from build123d import *

# Parameters (mm, degrees)
BOSS_EXTRUDE1_DEPTH        = 76.2
SKETCH2_R                  = 38.1
BOSS_EXTRUDE2_DEPTH        = 12.7
F_3_4_1_5_DIAMETER_HOLE1_D = 38.1


with BuildPart() as part:
    # Sketch1 → Boss-Extrude1 (new body)
    with BuildSketch(Plane.XY):
        with BuildLine():
            ThreePointArc((0, 74.498522628), (-11.550198291, 75.086541233), (-18.788031752, 66.066196825))
            Line((-18.788031752, 66.066196825), (-31.095079379, 6.415492062))
            ThreePointArc((-31.095079379, 6.415492062), (-24.614572645, -20.054558422), (0, -31.75))
            Line((0, -31.75), (19.05, -31.75))
            Line((19.05, -31.75), (19.05, -44.45))
            Line((19.05, -44.45), (88.9, -44.45))
            Line((88.9, -44.45), (114.3, -25.4))
            Line((114.3, -25.4), (114.3, -12.7))
            Line((114.3, -12.7), (50.8, -12.7))
            Line((50.8, -12.7), (50.8, 0))
            Line((50.8, 0), (0, 0))
            Line((0, 0), (0, 74.498522628))
        make_face()
    extrude(amount=BOSS_EXTRUDE1_DEPTH)

    # Sketch2 → Boss-Extrude2 (add)
    with BuildSketch(Plane(origin=(0, -12.7, 0), x_dir=(1, 0, 0), z_dir=(0, 1, 0))):
        with Locations((50.8, -38.1)):
            Circle(SKETCH2_R)
    extrude(amount=BOSS_EXTRUDE2_DEPTH)

    # 3/4 (1.5) Diameter Hole1 (through all)
    with Locations(Plane(origin=(0, 0, 0), x_dir=(1, 0, 0), z_dir=(0, 1, 0))):
        with Locations((50.8, -38.1)):
            Hole(F_3_4_1_5_DIAMETER_HOLE1_D / 2)


solid = part.part
Could you check a few things on this model? Use its own coordinates, in mm. A direction names the side the tool comes from. Coordinates: 2 decimals unless noted, no trailing zeros. Order: outer loops, then holes, each group sorted by start corner. A loop starts at its lowest first (then second) coordinate and runs counter-clockwise, first axis right, second up. Notation, with made-up numbers: (17, -39.5) - (70, -39.5) arc R21 ccw to (70, -32.5) - close; hole circle Ø9 at (71, 25.25). An arc over 180 degrees is marked (long way). Answer in a Markdown table with one row per item. Add a question column.
(1) Will these pins go through, and if not, where does the flat tip stop? pin 1 (23 mm diameter, centred on x = 50.8, z = 38.1, fed in from -Y); pin 2 (5.5 mm diameter, centred on x = 9.5, z = 36, fed in from -Y); pin 3 (12 mm diameter, centred on x = 72.5, y = 1.5, fed in from +Z); pin 4 (3 mm diameter, centred on x = 20, z = 21, fed in from +Y).
(2) On a 3-axis mill with a long thin cutter (end or side, diameter ignored), from which of +Z, -Z, +X, -X, +Y, -Y can I reach the whole of each face in a straight line? I mean faces 4 (the face through (9, -31.75, 38)), 5 (the face through (0, 37, 38)), 6 (the face through (69, -44.45, 46)). Say none if no direction works.
(3) If we section it at D-D, the plane y = 22.5: Please give me the cut outline in (x, z), then the cut area to 3 significant figures.
(4) If we section it at A-A, the plane z = 38.1: Please give me the cut outline in (x, y).
(5) I need wall thicknesses on L1, parallel to Z at x = 50.8, y = -23; L2, parallel to Y at x = 12, z = 21; L3, parallel to Y at x = 65, z = 16.5. Which ranges of each line are inside material? Lowest first, please.
(6) If we section it at B-B, the plane x = 4.5: Please give me the cut outline in (y, z), then the cut area to 3 significant figures.
(7) If we mould it in two halves opening along Z, with no side actions, what happens to faces 1 (the face through (88.89, -6.44, 38.94)), 2 (the face through (-24.855, 36.658, 37.567)), 3 (the face through (40.559, -22.536, 22.037))? For each: released by +Z, released by -Z, zero draft, split by the parting line, or undercut.
(8) If we section it at C-C, the plane z = 49: Please give me the cut outline in (x, y).
Results are:
| question | item | result |
|---|---|---|
| 1 | pin 1 | passes through |
| 1 | pin 2 | stops at y = -31.75 |
| 1 | pin 3 | stops at z = 72.73 |
| 1 | pin 4 | stops at y = 0 |
| 2 | face 4 | +Z, -Z, -X, -Y |
| 2 | face 5 | +Z, -Z, +X, +Y |
| 2 | face 6 | +Z, -Z, +X, -X, -Y |
| 3 | outline | (-27.78, 0) - (0, 0) - (0, 76.2) - (-27.78, 76.2) - close |
| 3 | area | 2,120 mm2 |
| 4 | outline | (-31.1, 6.42) arc R31.75 ccw to (0, -31.75) - (19.05, -31.75) - (19.05, -44.45) - (31.75, -44.45) - (31.75, 0) - (0, 0) - (0, 74.5) arc R12.7 ccw to (-18.79, 66.07) - close; (69.85, -44.45) - (88.9, -44.45) - (114.3, -25.4) - (114.3, -12.7) - (88.9, -12.7) - (88.9, 0) - (69.85, 0) - close |
| 5 | L1 | z = 0 to 19.05, 57.15 to 76.2 |
| 5 | L2 | y = -31.75 to 0 |
| 5 | L3 | y = -44.45 to 0 |
| 6 | outline | (-31.75, 0) - (0, 0) - (0, 76.2) - (-31.75, 76.2) - close |
| 6 | area | 2,420 mm2 |
| 7 | face 1 | split by the parting line |
| 7 | face 2 | zero draft |
| 7 | face 3 | undercut |
| 8 | outline | (-31.1, 6.42) arc R31.75 ccw to (0, -31.75) - (19.05, -31.75) - (19.05, -44.45) - (35.18, -44.45) - (35.18, 0) - (0, 0) - (0, 74.5) arc R12.7 ccw to (-18.79, 66.07) - close; (66.42, -44.45) - (88.9, -44.45) - (114.3, -25.4) - (114.3, -12.7) - (87.31, -12.7) - (87.31, 0) - (66.42, 0) - close |
